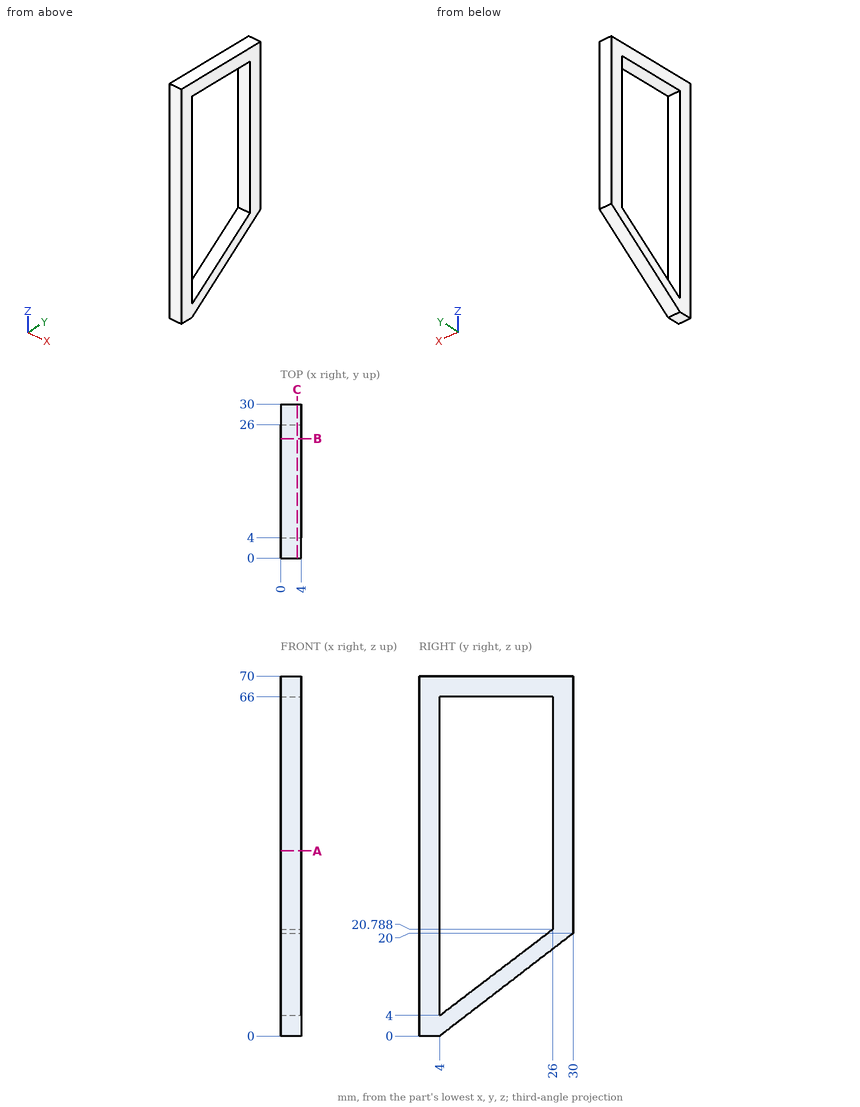
Check sheet for the drawn part. Datum: minimum x, y, z corner. Units: mm. Round coordinates to 2 decimals unless told otherwise and drop trailing zeros. Order: outer loops, then holes, each group sorted by start corner. A loop starts at its lowest first (then second) coordinate and runs counter-clockwise, first axis right, second up.
(1) Scan lines: probe 1 along Y at (x, z) = (1.4, 55.5); probe 2 along Z at (x, y) = (3.3, 7); probe 3 along Z at (x, y) = (1.2, 5.5) (1 decimal). Record each from-to range of solid material in increasing order.
(2) Cross-section at C-C, the plane x = 3.2. Enter the section's corners in (y, z).
(3) Cross-section at A-A, the plane z = 36. Enter the section's corners in (x, y), and give its area (3 significant figures).
(4) Cross-section at B-B, the plane y = 23.25. Enter the section's corners in (x, z).
Check sheet entries:
1. probe 1: y = 0 to 4, 26 to 30
1. probe 2: z = 2.31 to 6.29, 66 to 70
1. probe 3: z = 1.2 to 5.1, 66 to 70
2. outline: (0, 0) - (4, 0) - (30, 20) - (30, 70) - (0, 70) - close; hole (4, 4) - (26, 20.79) - (26, 66) - (4, 66) - close
3. outline: (0, 0) - (4, 0) - (4, 4) - (0, 4) - close; (0, 26) - (4, 26) - (4, 30) - (0, 30) - close
3. area: 32.0 mm2
4. outline: (0, 14.81) - (4, 14.81) - (4, 18.69) - (0, 18.69) - close; (0, 66) - (4, 66) - (4, 70) - (0, 70) - close
